from build123d import *

# Parameters (mm, degrees)
F0_R     = 3.175
F1_DEPTH = 1.905


with BuildPart() as f1:
    # F0 (on Front) → F1 (new body)
    with BuildSketch(Plane.XZ):
        with BuildLine():
            Line((-62.950969, -32.115153), (-62.950969, -34.147153))
            Line((-62.950969, -34.147153), (-35.963469, -34.147153))
            Line((-35.963469, -34.147153), (-35.963469, -36.179153))
            Line((-35.963469, -36.179153), (-23.263469, -36.179153))
            Line((-23.263469, -36.179153), (-23.301246, -34.147504))
            Line((-23.301246, -34.147504), (3.724031, -34.147504))
            Line((3.724031, -34.147504), (3.724031, -27.77421))
            ThreePointArc((3.724031, -27.77421), (0.930031, -24.622153), (3.724031, -21.470096))
            Line((3.724031, -21.470096), (3.724031, -18.24921))
            ThreePointArc((3.724031, -18.24921), (0.930031, -15.097153), (3.724031, -11.945096))
            Line((3.724031, -11.945096), (3.724031, -8.72421))
            ThreePointArc((3.724031, -8.72421), (0.930031, -5.572153), (3.724031, -2.420096))
            Line((3.724031, -2.420096), (3.724031, 0.80079))
            ThreePointArc((3.724031, 0.80079), (0.930031, 3.952847), (3.724031, 7.104904))
            Line((3.724031, 7.104904), (3.724031, 10.32579))
            ThreePointArc((3.724031, 10.32579), (0.930031, 13.477847), (3.724031, 16.629904))
            Line((3.724031, 16.629904), (3.724031, 19.85079))
            ThreePointArc((3.724031, 19.85079), (0.930031, 23.002847), (3.724031, 26.154904))
            Line((3.724031, 26.154904), (3.724031, 29.37579))
            ThreePointArc((3.724031, 29.37579), (1.355759, 30.939727), (1.184208, 33.772603))
            Line((1.184208, 33.772603), (-10.666718, 39.58069))
            ThreePointArc((-10.666718, 39.58069), (-14.029229, 39.188757), (-15.833969, 42.052847))
            Line((-15.833969, 42.052847), (-17.865969, 42.052847))
            ThreePointArc((-17.865969, 42.052847), (-21.040969, 38.877847), (-24.215969, 42.052847))
            Line((-24.215969, 42.052847), (-26.247969, 42.052847))
            ThreePointArc((-26.247969, 42.052847), (-29.422969, 38.877847), (-32.597969, 42.052847))
            Line((-32.597969, 42.052847), (-34.629969, 42.052847))
            ThreePointArc((-34.629969, 42.052847), (-37.804969, 38.877847), (-40.979969, 42.052847))
            Line((-40.979969, 42.052847), (-43.011969, 42.052847))
            ThreePointArc((-43.011969, 42.052847), (-44.899665, 39.150525), (-48.318094, 39.699354))
            Line((-48.318094, 39.699354), (-60.099957, 33.925115))
            ThreePointArc((-60.099957, 33.925115), (-60.256813, 30.847922), (-62.950969, 29.352847))
            Line((-62.950969, 29.352847), (-62.950969, 26.177847))
            ThreePointArc((-62.950969, 26.177847), (-59.775969, 23.002847), (-62.950969, 19.827847))
            Line((-62.950969, 19.827847), (-62.950969, 16.652847))
            ThreePointArc((-62.950969, 16.652847), (-59.775969, 13.477847), (-62.950969, 10.302847))
            Line((-62.950969, 10.302847), (-62.950969, 7.127847))
            ThreePointArc((-62.950969, 7.127847), (-59.775969, 3.952847), (-62.950969, 0.777847))
            Line((-62.950969, 0.777847), (-62.950969, -2.397153))
            ThreePointArc((-62.950969, -2.397153), (-59.775969, -5.572153), (-62.950969, -8.747153))
            Line((-62.950969, -8.747153), (-62.950969, -11.922153))
            ThreePointArc((-62.950969, -11.922153), (-59.775969, -15.097153), (-62.950969, -18.272153))
            Line((-62.950969, -18.272153), (-62.950969, -21.447153))
            ThreePointArc((-62.950969, -21.447153), (-59.775969, -24.622153), (-62.950969, -27.797153))
            Line((-62.950969, -27.797153), (-62.950969, -32.115153))
        make_face()
        with Locations((-54.568969, -24.622153)):
            Circle(F0_R, mode=Mode.SUBTRACT)
        with Locations((-46.186969, -24.622153)):
            Circle(F0_R, mode=Mode.SUBTRACT)
        with Locations((-37.804969, -24.622153)):
            Circle(F0_R, mode=Mode.SUBTRACT)
        with Locations((-54.568969, -15.097153)):
            Circle(F0_R, mode=Mode.SUBTRACT)
        with Locations((-54.568969, -5.572153)):
            Circle(F0_R, mode=Mode.SUBTRACT)
        with BuildLine():
            ThreePointArc((-47.838028, -12.385211), (-29.704319, 20.780156), (-11.292136, -12.231425))
            ThreePointArc((-11.292136, -12.231425), (-10.231083, -17.143124), (-15.251558, -16.929939))
            ThreePointArc((-15.251558, -16.929939), (-29.462073, -22.399122), (-43.747891, -17.129769))
            ThreePointArc((-43.747891, -17.129769), (-48.591745, -17.170236), (-47.838028, -12.385211))
        make_face(mode=Mode.SUBTRACT)
        with Locations((-21.040969, -24.622153)):
            Circle(F0_R, mode=Mode.SUBTRACT)
        with Locations((-12.658969, -24.622153)):
            Circle(F0_R, mode=Mode.SUBTRACT)
        with Locations((-4.276969, -24.622153)):
            Circle(F0_R, mode=Mode.SUBTRACT)
        with Locations((-4.276969, -15.097153)):
            Circle(F0_R, mode=Mode.SUBTRACT)
        with Locations((-4.276969, -5.572153)):
            Circle(F0_R, mode=Mode.SUBTRACT)
        with Locations((-54.568969, 3.952847)):
            Circle(F0_R, mode=Mode.SUBTRACT)
        with Locations((-54.568969, 13.477847)):
            Circle(F0_R, mode=Mode.SUBTRACT)
        with Locations((-54.568969, 23.002847)):
            Circle(F0_R, mode=Mode.SUBTRACT)
        with Locations((-54.568969, 32.527847)):
            Circle(F0_R, mode=Mode.SUBTRACT)
        with Locations((-46.186969, 23.002847)):
            Circle(F0_R, mode=Mode.SUBTRACT)
        with Locations((-37.804969, 23.002847)):
            Circle(F0_R, mode=Mode.SUBTRACT)
        with Locations((-46.186969, 32.527847)):
            Circle(F0_R, mode=Mode.SUBTRACT)
        with Locations((-37.804969, 32.527847)):
            Circle(F0_R, mode=Mode.SUBTRACT)
        with Locations((-4.276969, 3.952847)):
            Circle(F0_R, mode=Mode.SUBTRACT)
        with Locations((-4.276969, 13.477847)):
            Circle(F0_R, mode=Mode.SUBTRACT)
        with Locations((-21.040969, 23.002847)):
            Circle(F0_R, mode=Mode.SUBTRACT)
        with Locations((-29.422969, 32.527847)):
            Circle(F0_R, mode=Mode.SUBTRACT)
        with Locations((-21.040969, 32.527847)):
            Circle(F0_R, mode=Mode.SUBTRACT)
        with Locations((-12.658969, 23.002847)):
            Circle(F0_R, mode=Mode.SUBTRACT)
        with Locations((-4.276969, 23.002847)):
            Circle(F0_R, mode=Mode.SUBTRACT)
        with Locations((-12.658969, 32.527847)):
            Circle(F0_R, mode=Mode.SUBTRACT)
        with Locations((-4.276969, 32.527847)):
            Circle(F0_R, mode=Mode.SUBTRACT)
    extrude(amount=F1_DEPTH)


solid = f1.part
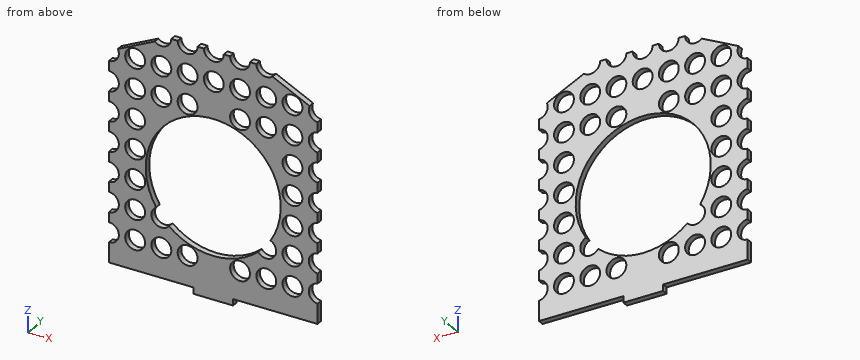
Check sheet for the modelled part. Datum: model origin and axes. Units: mm. Give positions to 0.01 mm unless a question says otherwise; leave off trailing zeros. Order: outer loops, then holes, each group sorted by start corner. A loop starts at its lowest first (then second) coordinate and runs counter-clockwise, first axis right, second up. Notation, with made-up numbers: (87, -9) - (127, -9) arc R28 cw to (127, 26) - close; hole circle Ø9 at (47.5, 65). An arc over 180 degrees is marked (long way). Answer as CSV lines item,"result".
1. Go/stop test with flat-tipped pins: P1, Ø4, axis at x = -4.28, z = -5.57, coming from the -Y side; P2, Ø10, axis at x = -54.57, z = -5.57, coming from the +Y side; P3, Ø1, axis at y = -0.5, z = 21, coming from the -X side. Record where each tip stops, or that it passes through.
Result sheet:
P1,"through"
P2,"y = 0"
P3,"x = -61"
2. Section check B-B (x = -30). Record the boundary of the cut face in (y, z) (3 decimals), then the cut area to 3 significant figures.
Result sheet:
outline,"(-1.905, -36.179) - (0, -36.179) - (0, -22.396) - (-1.905, -22.396) - close; (-1.905, 20.777) - (0, 20.777) - (0, 29.406) - (-1.905, 29.406) - close; (-1.905, 35.65) - (0, 35.65) - (0, 38.931) - (-1.905, 38.931) - close"
area,"48.9 mm²"
3. Scan lines: probe 1 along Z at (x, y) = (-11.5, -1.45); probe 2 along Z at (x, y) = (-47.5, -1.2); probe 3 along Z at (x, y) = (-31, -0.15). Record each from-to range of solid material in increasing order. Write a range as from..to.
Result sheet:
probe 1,"-34.15..-27.58, -21.67..-18.05, 10.94..20.05, 25.96..29.57, 35.48..39.1"
probe 2,"-34.15..-27.51, -21.73..-17.99, 11.28..20.11, 25.89..29.64, 35.42..39.16"
probe 3,"-36.18..-22.36, 20.74..29.77, 35.28..39.3"
4. Section check A-A (z = 15.5). Record the boundary of the cut face in (x, y) (3 decimals).
Result sheet:
outline,"(-60.503, -1.905) - (-57.017, -1.905) - (-57.017, 0) - (-60.503, 0) - close; (-52.121, -1.905) - (-43.76, -1.905) - (-43.76, 0) - (-52.121, 0) - close; (-15.467, -1.905) - (-6.725, -1.905) - (-6.725, 0) - (-15.467, 0) - close; (-1.829, -1.905) - (1.657, -1.905) - (1.657, 0) - (-1.829, 0) - close"
5. Section check C-C (x = -2.5). State how many separate pieces and enclosed holes the cut face has, then the cut area to 3 significant figures.
Result sheet:
separate pieces,"8"
enclosed holes,"0"
area,"62.7 mm²"
6. Section check D-D (x = -12.5). Record the boundary of the cut face in (y, z) (1 decimal).
Result sheet:
outline,"(-1.9, -34.1) - (0, -34.1) - (0, -27.8) - (-1.9, -27.8) - close; (-1.9, -21.5) - (0, -21.5) - (0, -18.3) - (-1.9, -18.3) - close; (-1.9, 12.4) - (0, 12.4) - (0, 19.8) - (-1.9, 19.8) - close; (-1.9, 26.2) - (0, 26.2) - (0, 29.4) - (-1.9, 29.4) - close; (-1.9, 35.7) - (0, 35.7) - (0, 38.9) - (-1.9, 38.9) - close"
